```python
from build123d import *

# Parameters (mm, degrees)
F0_W     = 114.3
F0_H     = 25.4
F1_DEPTH = 50.165
F2_R     = 7.493
F3_DEPTH = 25.4
F4_R     = 2.5527
F5_DEPTH = 25.4
F7_DEPTH = 5.5626


with BuildPart() as f1:
    # F0 (on Top) → F1 (new body)
    with BuildSketch(Plane.XY):
        with Locations((57.15, 12.7)):
            Rectangle(F0_W, F0_H)
    extrude(amount=F1_DEPTH)

    # F2 (on face) → F3 (cut)
    with BuildSketch(Plane.XZ):
        with Locations((47.625, 32.512)):
            Circle(F2_R)
    extrude(amount=-F3_DEPTH, mode=Mode.SUBTRACT)

    # F4 (on face) → F5 (cut)
    with BuildSketch(Plane(origin=(0, 0, 0), x_dir=(1, 0, 0), z_dir=(0, 0, -1))):
        with Locations((19.05, -12.7)):
            Circle(F4_R)
        with Locations((95.25, -12.7)):
            Circle(F4_R)
    extrude(amount=-F5_DEPTH, mode=Mode.SUBTRACT)

    # F6 (on face) → F7 (cut)
    with BuildSketch(Plane(origin=(0, 0, 0), x_dir=(1, 0, 0), z_dir=(0, 0, -1))):
        Polygon((12.634195, -12.7), (15.842098, -18.25625), (22.257902, -18.25625), (25.465805, -12.7), (22.257902, -7.14375), (15.842098, -7.14375), align=None)
        Polygon((88.834195, -12.7), (92.042098, -18.25625), (98.457902, -18.25625), (101.665805, -12.7), (98.457902, -7.14375), (92.042098, -7.14375), align=None)
    extrude(amount=-F7_DEPTH, mode=Mode.SUBTRACT)


solid = f1.part
```
Geometry: final body of the model. Coordinates: model frame, mm. A direction names the side the tool comes from. Give positions to 0.01 mm unless a question says otherwise; leave off trailing zeros. Write each loop counter-clockwise with the first axis right and the second up, starting at its lowest first coordinate (ties: lowest second). Pieces come first, ordered by that corner, then holes.
1. Draft query along Y for faces 1 (the cylindrical face through (41.68, 12.52, 27.95)), 2 (the flat face through (56, 0, 25)), 3 (the flat face through (14.216, 15.439, 2.742)), 4 (the flat face through (19, 13, 25.4)). Return one class per face: released by +Y, released by -Y, zero draft, split by the parting line, or undercut.
2. Section query D-D, the plane y = 21. Return loops of the section in (x, z) (3 decimals), then the cut area to 3 significant figures.
3. Line query: probe 1 along X at (y, z) = (12.7, 16.75); probe 2 along Y at (x, z) = (19, 10); probe 3 along X at (y, z) = (15, 8). Output: solid intervals per line, ascending.
4. Pin query (flat end, axial travel): P1, Ø3.5, axis at x = 16.5, y = 10.5, coming from the -Z side; P2, Ø4, axis at x = 19.05, y = 12.7, coming from the -Z side. Return the tip coordinate at first contact, or that it passes through.
5. Section query B-B, the plane x = 95.25. Return loops of the section in (y, z) (3 decimals).
6. Reachability of faces 5 (the flat face through (90.461, 9.883, 2.742)), 6 (the flat face through (0, 13, 25)) from +Z, -Z, +X, -X, +Y, -Y: full face, straight path, thin tool, end or side. Return the list, or none.
7. Section query C-C, the plane z = 38. Return loops of the section in (x, y), then the cut area to 3 significant figures.
8. Section query A-A, the plane z = 3. Return loops of the section in (x, y).
Computed:
1. face 1: zero draft
1. face 2: released by -Y
1. face 3: undercut
1. face 4: undercut
2. outline: (0, 0) - (114.3, 0) - (114.3, 50.165) - (0, 50.165) - close; hole circle Ø14.986 at (47.625, 32.512)
2. area: 5,560 mm2
3. probe 1: x = 0 to 16.5, 21.6 to 92.7, 97.8 to 114.3
3. probe 2: y = 0 to 10.15, 15.25 to 25.4
3. probe 3: x = 0 to 17.94, 20.16 to 94.14, 96.36 to 114.3
4. P1: stops at z = 5.56
4. P2: stops at z = 25.4
5. outline: (0, 0) - (7.144, 0) - (7.144, 5.563) - (10.147, 5.563) - (10.147, 25.4) - (15.253, 25.4) - (15.253, 5.563) - (18.256, 5.563) - (18.256, 0) - (25.4, 0) - (25.4, 50.165) - (0, 50.165) - close
6. face 5: -Z
6. face 6: +Z, -Z, -X, +Y, -Y
7. outline: (0, 0) - (42.52, 0) - (42.52, 25.4) - (0, 25.4) - close; (52.73, 0) - (114.3, 0) - (114.3, 25.4) - (52.73, 25.4) - close
7. area: 2,640 mm2
8. outline: (0, 0) - (114.3, 0) - (114.3, 25.4) - (0, 25.4) - close; hole (12.63, 12.7) - (15.84, 7.14) - (22.26, 7.14) - (25.47, 12.7) - (22.26, 18.26) - (15.84, 18.26) - close; hole (88.83, 12.7) - (92.04, 7.14) - (98.46, 7.14) - (101.67, 12.7) - (98.46, 18.26) - (92.04, 18.26) - close
